Could you check a few things on this model? Use its own coordinates, in mm. Face numbers are marked on the shaded views. Round coordinates to 2 decimals unless told otherwise and drop trailing zeros. Write each loop counter-clockwise with the first axis right and the second up, starting at its lowest first coordinate (ties: lowest second). Pieces come first, ordered by that corner, then holes. Notation, with made-up numbers: (-24, -15.75) -> (4, -15.75) arc R26 cw to (4, 21.25) -> close; hole circle Ø8 at (60, 6.5). An arc over 180 degrees is marked (long way). Return JSON: item names as keys, results as strings.
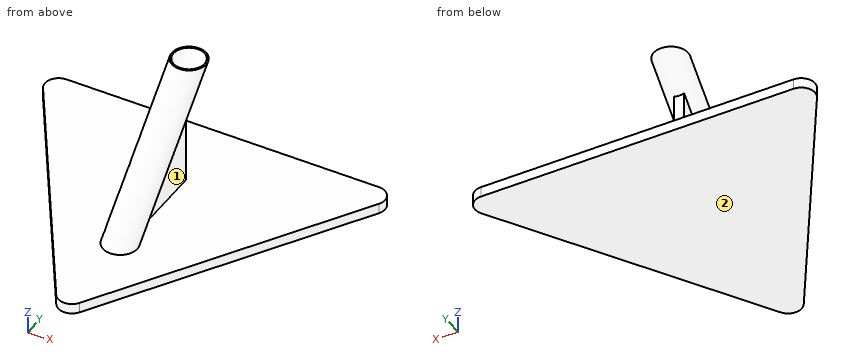
from build123d import *

# Parameters (mm, degrees)
BOSS_EXTRU_1_DEPTH = 3
ESQUISSE5_R        = 5
ESQUISSE7_R        = 4.5
NERVURE4_REACH     = 109.103
ESQUISSE10_WALL_W  = 242.432835572
ESQUISSE10_WALL_H  = 3
CONG_1_R           = 4


with BuildPart() as part:
    # Esquisse1 → Boss.-Extru.1 (new body)
    with BuildSketch(Plane.XY):
        Polygon((0, 0), (-52.726441393, 84.970126386), (52.726441393, 84.970126386), align=None)
    extrude(amount=BOSS_EXTRU_1_DEPTH)

    # Balayage1: sweep along a path in Esquisse6
    with BuildLine(Plane(origin=(0, 0, 0), x_dir=(0, 0, -1), z_dir=(1, 0, 0))) as balayage1_path:
        Line((-3, 32.30290769), (-38.355339059, 67.65824675))
    # Esquisse5 → Balayage1 (sweep)
    with BuildSketch(Plane.XY.offset(3)):
        with Locations((0, 32.30290769)):
            Circle(ESQUISSE5_R)
    sweep(path=balayage1_path.line)

    # Enlèvement de matière-Balayage1: sweep along a path in Esquisse6<2>
    with BuildLine(Plane(origin=(0, 0, 0), x_dir=(0, 0, -1), z_dir=(1, 0, 0))) as enl_vement_de_mati_re_balayage1_path:
        Line((-3, 32.30290769), (-38.355339059, 67.65824675))
    # Esquisse7 → Enlèvement de matière-Balayage1 (sweep, cut)
    with BuildSketch(Plane.XY.offset(3)):
        with Locations((0, 32.30290769)):
            Circle(ESQUISSE7_R)
    sweep(path=enl_vement_de_mati_re_balayage1_path.line, mode=Mode.SUBTRACT)

    # Esquisse10 wall → Nervure4 (add, up to next)
    with BuildSketch(Plane(origin=(0, 63.529001685, 16.113046997), x_dir=(0, 0, -1), z_dir=(0, 1, 0)), mode=Mode.PRIVATE) as nervure4_sk1:
        Rectangle(ESQUISSE10_WALL_W, ESQUISSE10_WALL_H)
    nervure4_tool1 = extrude(nervure4_sk1.sketch, amount=-NERVURE4_REACH, mode=Mode.PRIVATE) - part.part
    add(nervure4_tool1.solids().sort_by_distance((0, 63.529001685, 16.113046997))[0])

    # Congé1
    cong_1_edges = [part.edges().sort_by_distance(p)[0] for p in [
        (0, 0, 1.5),
        (-52.726441393, 84.970126386, 1.5),
        (52.726441393, 84.970126386, 1.5),
    ]]
    fillet(cong_1_edges, radius=CONG_1_R)


solid = part.part
1) Will these pins go through, and if not, where does the flat tip stop? pin 1 Ø3 at (x, z) = (-2.5, 22) entering from -Y; pin 2 Ø1.5 at (x, z) = (0, 21) entering from +Y; pin 3 Ø2.5 at (x, y) = (-1.5, 33) entering from +Z.
Return value:
{"pin 1": "y = 45.3", "pin 2": "y = 63.53", "pin 3": "z = 9.76"}
2) If I drill on probe 1 along Z at (x, y) = (28, 56); probe 2 along X at (y, z) = (42, 5); probe 3 along Y at (x, z) = (0.5, 11), over which ranges is the centre line in solid material (lowest first)? Write a range as [from, to].
Return value:
{"probe 1": "[0, 3]", "probe 2": "[-1.5, 1.5]", "probe 3": "[35.33, 35.83], [44.78, 63.53]"}
3) Thinking about a two-plate mould opening in Z: for the marked faces 1 and 2, which applies, pulls with the +Z half, pulls with the -Z half, needs draft (parallel to the pull), parting line crosses it, or undercut?
Return value:
{"face 1": "undercut", "face 2": "pulls with the -Z half"}
4) I want a section at A-A, the plane y = 17. Please give me the cut outline in (x, z).
Return value:
{"outline": "(-10.55, 0) -> (10.55, 0) -> (10.55, 3) -> (-10.55, 3) -> close"}
5) I want a section at B-B, the plane x = -13. Please give me the cut outline in (y, z).
Return value:
{"outline": "(20.95, 0) -> (84.97, 0) -> (84.97, 3) -> (20.95, 3) -> close"}
